Can you work these out from the model? Positions are in its coordinate system, mm. A direction names the side the tool comes from. Round coordinates to 2 decimals unless told otherwise and drop trailing zeros. Loops run counter-clockwise (first coordinate to the right, second up) from the corner with the lowest first, then second, coordinate; pieces in that order, holes last. Notation, with made-up numbers: (46, -40) -> (55, -40) arc R27 ccw to (55, -1) -> close; hole circle Ø6 at (25, 13.25). An arc over 180 degrees is marked (long way). Write item = value, one per line.
from build123d import *


with BuildPart() as part:
    # Esquisse1 → Révolution1 (revolve)
    with BuildSketch(Plane.XY, mode=Mode.PRIVATE) as r_volution1_sk:
        Polygon((-28.565758671, 25.213681359), (-18.565758671, 25.213681359), (-18.565758671, 26.213681359), (-13.565758671, 26.213681359), (31.434241329, 8.213681359), (31.434241329, 5.213681359), (-15.565758671, 5.213681359), (-15.565758671, 7.213681359), (-28.565758671, 7.213681359), align=None)
    revolve(r_volution1_sk.sketch.rotate(Axis((-43.545779604, -13.286318641, 0), (1, 0, 0)), 90), axis=Axis((-43.545779604, -13.286318641, 0), (1, 0, 0)))  # turned: the seam where the file's is


solid = part.part
1. I'm going to push flat-ended pins straight in: pin 1 (12 mm diameter, centred on x = 8.5, y = -21.5, fed in from +Z); pin 2 (4 mm diameter, centred on x = -14, z = 28, fed in from -Y); pin 3 (3 mm diameter, centred on x = -6, y = -10, fed in from +Z). Where does each tip first touch, or does it pass through?
Entries:
pin_1 = 32.36
pin_2 = -43.02
pin_3 = 36.94
2. For faces 1 (the conical face through (19.25, 10.11, 12.17)), 2 (the flat face through (-18.566, -5, -38)), which set-ups out of +Z, -Z, +X, -X, +Y, -Y let a thin tool reach every point of the face, with its end or its side?
Entries:
face_1 = +X
face_2 = -X
3. Suppose I cut it at A-A, the plane z = 0. List the corners of the cut face in (x, y) for me, and give its area (3 significant figures).
Entries:
outline = (-28.57, -51.79) -> (-18.57, -51.79) -> (-18.57, -52.79) -> (-13.57, -52.79) -> (31.43, -34.79) -> (31.43, -31.79) -> (-15.57, -31.79) -> (-15.57, -33.79) -> (-28.57, -33.79) -> close; (-28.57, 7.21) -> (-15.57, 7.21) -> (-15.57, 5.21) -> (31.43, 5.21) -> (31.43, 8.21) -> (-13.57, 26.21) -> (-18.57, 26.21) -> (-18.57, 25.21) -> (-28.57, 25.21) -> close
area = 1,640 mm²
4. I need wall thicknesses on line 1 (Y direction, x = -18.75, z = 0); line 2 (Z direction, x = 10.5, y = -8.5); line 3 (Y direction, x = 4, z = 0). Which ranges of each line are inside material? Lowest first, please. Write a range as [from, to].
Entries:
line_1 = [-51.79, -33.79], [7.21, 25.21]
line_2 = [-29.49, -17.87], [17.87, 29.49]
line_3 = [-45.76, -31.79], [5.21, 19.19]
5. We'd pull the mould along Z, two halves only. Please class faces 3 (the cylindrical face through (-16.031, -39.982, -29.113)), 4 (the cylindrical face through (7.605, 4.774, -4.01)), 5 (the flat face through (31.434, -31, 6)): released by +Z, released by -Z, zero draft, split by the parting line, or undercut.
Entries:
face_3 = split by the parting line
face_4 = undercut
face_5 = zero draft
6. Suppose I cut it at C-C, the plane x = -21. List the corners of the cut face in (y, z) for me.
Entries:
outline = circle Ø77 at (-13.29, 0); hole circle Ø41 at (-13.29, 0)
7. Suppose I cut it at B-B, the plane x = 27.5. List the corners of the cut face in (y, z) for me.
Entries:
outline = circle Ø46.15 at (-13.29, 0); hole circle Ø37 at (-13.29, 0)
